Read the model definition and answer for the solid it produces. Units are mm, in the model's axes. Coordinates: 2 decimals unless noted, no trailing zeros. Write each loop counter-clockwise with the first axis right and the second up, starting at its lowest first coordinate (ties: lowest second). Pieces come first, ordered by that corner, then holes.
1) The part is cut by section D-D (z = -7). Determine the outline of the cut face in (x, y).
2) The part is cut by section B-B (x = 75). Determine the outline of the cut face in (y, z), then the cut area to 3 significant figures.
3) The part is cut by section A-A (y = 0.7). Determine the outline of the cut face in (x, z).
4) The part is cut by section C-C (z = -4). Determine the outline of the cut face in (x, y), then the cut area to 3 significant figures.
5) Each of these flat-tipped pins is pushed along its axis until it touches: pin 1 Ø1 at (x, y) = (6, 0.5) entering from -Z; pin 2 Ø4 at (x, z) = (19, -13) entering from -Y (3 decimals); pin 3 Ø1 at (x, y) = (49.5, 1) entering from +Z. Where does it stop, or does it pass through?
6) Find the intervals of material crossed by line 1 (X direction, y = 1.3, z = -2.5); line 2 (X direction, y = 0.9, z = -8.75); line 3 (X direction, y = 0.6, z = -8.5), in increasing order.
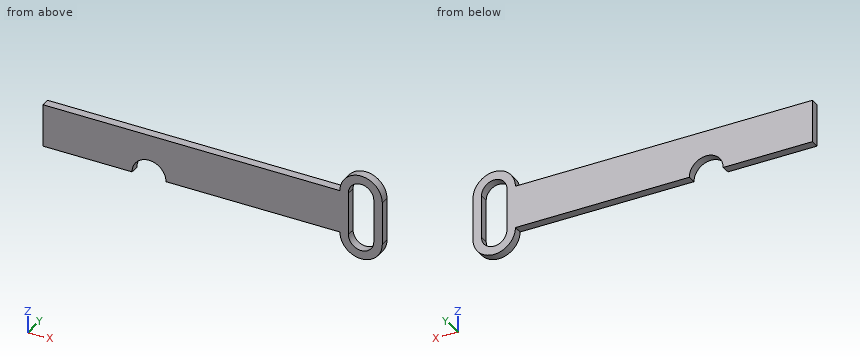
from build123d import *

# Parameters (mm, degrees)
BOSS_EXTRUDE1_DEPTH = 2
BOSS_EXTRUDE2_DEPTH = 2
CUT_EXTRUDE1_DEPTH  = 2


with BuildPart() as part:
    # Sketch1 → Boss-Extrude1 (new body)
    with BuildSketch(Plane(origin=(0, 0, 0), x_dir=(1, 0, 0), z_dir=(0, 1, 0))):
        with BuildLine():
            Line((0, 10), (0, 0))
            Line((0, 0), (70, 0))
            Line((70, 0), (70, 10))
            Line((70, 10), (29, 10))
            ThreePointArc((29, 10), (25, 6), (21, 10))
            Line((21, 10), (0, 10))
        make_face()
    extrude(amount=BOSS_EXTRUDE1_DEPTH)

    # Sketch2 → Boss-Extrude2 (add)
    with BuildSketch(Plane(origin=(0, 2, 0), x_dir=(1, 0, 0), z_dir=(0, 1, 0))):
        with BuildLine():
            Line((80, 10), (80, 0))
            ThreePointArc((80, 0), (75, -5), (70, 0))
            Line((70, 0), (70, 10))
            ThreePointArc((70, 10), (75, 15), (80, 10))
        make_face()
    extrude(amount=-BOSS_EXTRUDE2_DEPTH)

    # Sketch3 → Cut-Extrude1 (cut)
    with BuildSketch(Plane(origin=(0, 2, 0), x_dir=(1, 0, 0), z_dir=(0, 1, 0))):
        with BuildLine():
            Line((78, 10), (78, 0))
            ThreePointArc((78, 0), (75, -3), (72, 0))
            Line((72, 0), (72, 10))
            ThreePointArc((72, 10), (75, 13), (78, 10))
        make_face()
    extrude(amount=-CUT_EXTRUDE1_DEPTH, mode=Mode.SUBTRACT)


solid = part.part
Reported:
1. outline: (0, 0) - (22.35, 0) - (22.35, 2) - (0, 2) - close; (27.65, 0) - (72, 0) - (72, 2) - (27.65, 2) - close; (78, 0) - (80, 0) - (80, 2) - (78, 2) - close
2. outline: (0, -15) - (2, -15) - (2, -13) - (0, -13) - close; (0, 3) - (2, 3) - (2, 5) - (0, 5) - close
2. area: 8.00 mm2
3. outline: (0, -10) - (21, -10) arc R4 cw to (29, -10) - (70, -10) arc R5 ccw to (80, -10) - (80, 0) arc R5 ccw to (70, 0) - (0, 0) - close; hole (72, -10) arc R3 ccw to (78, -10) - (78, 0) arc R3 ccw to (72, 0) - close
4. outline: (0, 0) - (72, 0) - (72, 2) - (0, 2) - close; (78, 0) - (80, 0) - (80, 2) - (78, 2) - close
4. area: 148 mm2
5. pin 1: stops at z = -10
5. pin 2: passes through
5. pin 3: stops at z = 0
6. line 1: x = 0 to 72, 78 to 80
6. line 2: x = 0 to 21.2, 28.8 to 72, 78 to 80
6. line 3: x = 0 to 21.29, 28.71 to 72, 78 to 80
